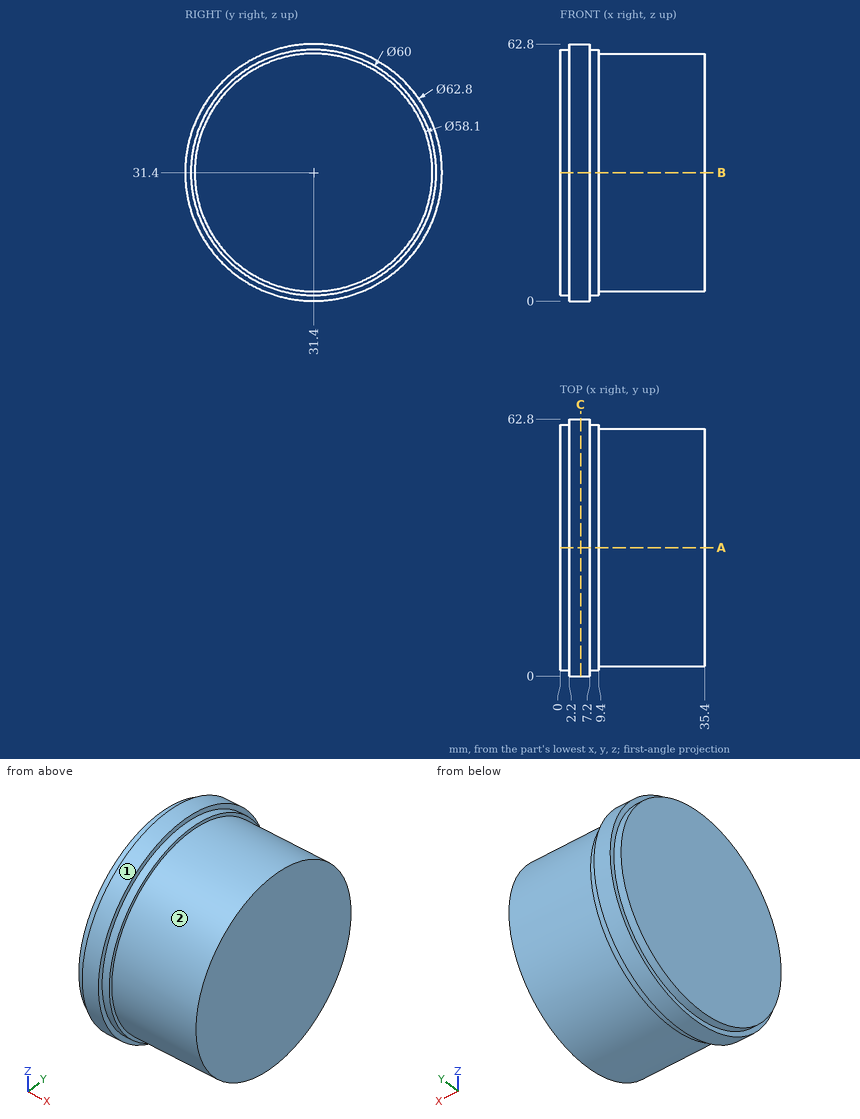
Job drawing, mm, ordinate dimensions from the low corner. One solid piece. A direction names the side the tool comes from. Coordinates: 2 decimals unless noted, no trailing zeros. Loops run counter-clockwise (first coordinate to the right, second up) from the corner with the lowest first, then second, coordinate; pieces in that order, holes last. Notation, with made-up numbers: (-21.5, 58.5) - (-13.5, 58.5) arc R15 ccw to (-13.5, 70.5) - close; hole circle Ø3 at (-36, 88). An arc over 180 degrees is marked (long way). Answer as a JSON object with one key per item and string values. Group by question number.
(1) Tool access for the marked faces 1 and 2: list every direction of +Z, -Z, +X, -X, +Y, -Y with a clear straight run to the whole face (end or side of a thin tool).
(2) Flat gauge pins, fed straight in: pin 1 (2 mm diameter, centred on x = 28, y = 56, fed in from -Z); pin 2 (5 mm diameter, centred on x = 4, z = 12.5, fed in from -Y); pin 3 (3 mm diameter, centred on x = 7, z = 27, fed in from +Y). Where does each tip first touch, or does it go through?
(3) Cut at A-A (y = 31.4). Give the cut face in (x, z).
(4) Cut at C-C (x = 5). Give the cut face in (y, z), then the cut area to 3 significant figures.
(5) Probe line 1 along Y through (x, z) = (27, 31); line 2 along X through (y, z) = (7, 49); line 3 along Z through (x, y) = (27.5, 14.5). List the from-to ranges inside material, lowest first.
Geometry says:
{
 "1": {"face 1": "+X, -X", "face 2": "+X"},
 "2": {"pin 1": "stops at z = 14.46", "pin 2": "stops at y = 4.62", "pin 3": "stops at y = 62.67"},
 "3": {"outline": "(0, 1.4) - (2.2, 1.4) - (2.2, 0) - (7.2, 0) - (7.2, 1.4) - (9.4, 1.4) - (9.4, 2.35) - (35.4, 2.35) - (35.4, 60.45) - (9.4, 60.45) - (9.4, 61.4) - (7.2, 61.4) - (7.2, 62.8) - (2.2, 62.8) - (2.2, 61.4) - (0, 61.4) - close"},
 "4": {"outline": "circle Ø62.8 at (31.4, 31.4)", "area": "3,100 mm^2"},
 "5": {"line 1": "y = 2.35 to 60.45", "line 2": "x = 2.2 to 7.2", "line 3": "z = 7.77 to 55.03"}
}
